Build history of the part. All positions in model axes, mm. Give positions to 0.01 mm unless a question says otherwise; leave off trailing zeros. Order: outer loops, then holes, each group sorted by start corner. A loop starts at its lowest first (then second) coordinate and runs counter-clockwise, first axis right, second up. Notation, with made-up numbers: (51, -37) - (63, -37) arc R27 ccw to (63, -13) - close; hole circle Ø11 at (45, -31). An arc over 180 degrees is marked (long way). Answer in a Markdown table with one row per item.
```python
from build123d import *

# Parameters (mm, degrees)
CROQUIS1_W              = 37
CROQUIS1_H              = 55
CROQUIS1_R              = 1.6
SALIENTE_EXTRUIR1_DEPTH = 2
REDONDEO1_R             = 5


with BuildPart() as part:
    # Croquis1 → Saliente-Extruir1 (new body)
    with BuildSketch(Plane(origin=(0, 0, 0), x_dir=(1, 0, 0), z_dir=(0, 1, 0))):
        Rectangle(CROQUIS1_W, CROQUIS1_H)
        with Locations((-13.5, 22.5)):
            Circle(CROQUIS1_R, mode=Mode.SUBTRACT)
        with Locations((-13.5, 2)):
            Circle(CROQUIS1_R, mode=Mode.SUBTRACT)
        with Locations((13.5, 2)):
            Circle(CROQUIS1_R, mode=Mode.SUBTRACT)
        with Locations((13.5, 22.5)):
            Circle(CROQUIS1_R, mode=Mode.SUBTRACT)
    extrude(amount=SALIENTE_EXTRUIR1_DEPTH)

    # Redondeo1
    redondeo1_edges = [part.edges().sort_by_distance(p)[0] for p in [
        (18.5, 1, 27.5),
        (-18.5, 1, 27.5),
        (-18.5, 1, -27.5),
        (18.5, 1, -27.5),
    ]]
    fillet(redondeo1_edges, radius=REDONDEO1_R)


solid = part.part
```
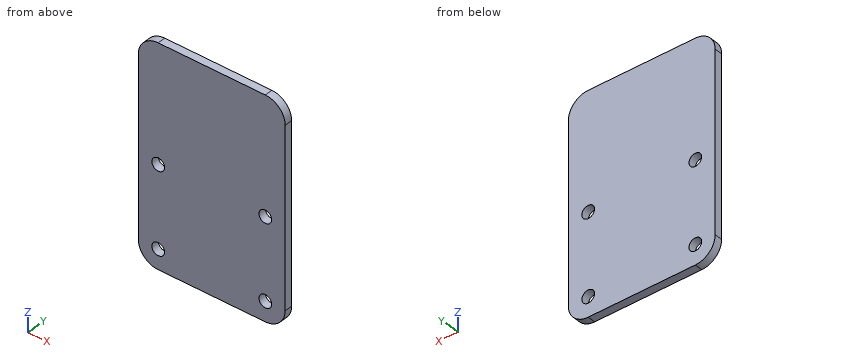
1. Cut at A-A on y = 0.7. Write the cut outline in (x, z), and give its area (3 significant figures).
Check result:
| item | result |
|---|---|
| outline | (-18.5, -22.5) arc R5 ccw to (-13.5, -27.5) - (13.5, -27.5) arc R5 ccw to (18.5, -22.5) - (18.5, 22.5) arc R5 ccw to (13.5, 27.5) - (-13.5, 27.5) arc R5 ccw to (-18.5, 22.5) - close; hole circle Ø3.2 at (-13.5, -22.5); hole circle Ø3.2 at (-13.5, -2); hole circle Ø3.2 at (13.5, -22.5); hole circle Ø3.2 at (13.5, -2) |
| area | 1,980 mm² |
2. Drop a flat-ended pin along its axis: P1, Ø1.9, axis at x = 13.5, z = -22.5, coming from the -Y side. Give the stop position or say it passes through.
Check result:
| item | result |
|---|---|
| P1 | passes through |
3. Cut at B-B on z = -2. Write the cut outline in (x, y).
Check result:
| item | result |
|---|---|
| outline | (-18.5, 0) - (-15.1, 0) - (-15.1, 2) - (-18.5, 2) - close; (-11.9, 0) - (11.9, 0) - (11.9, 2) - (-11.9, 2) - close; (15.1, 0) - (18.5, 0) - (18.5, 2) - (15.1, 2) - close |
4. Probe line 1 (X direction, y = 1.25, z = -2); line 2 (Z direction, x = -13.5, y = 0.8); line 3 (Z direction, x = 12.5, y = 0.3). List the from-to ranges inside material, lowest first.
Check result:
| item | result |
|---|---|
| line 1 | x = -18.5 to -15.1, -11.9 to 11.9, 15.1 to 18.5 |
| line 2 | z = -27.5 to -24.1, -20.9 to -3.6, -0.4 to 27.5 |
| line 3 | z = -27.5 to -23.75, -21.25 to -3.25, -0.75 to 27.5 |
